from build123d import *

# Parameters (mm, degrees)
F0_R          = 15
F1_DEPTH      = 13
F3_DEPTH      = 25
F3_DEPTH_BACK = 10
F4_R          = 1.5
F5_DEPTH      = 13.001


with BuildPart() as f1:
    # F0 (on Top) → F1 (new body)
    with BuildSketch(Plane.XY):
        Circle(F0_R)
    extrude(amount=F1_DEPTH)

    # F2 (on Right) → F3 (cut, two sides)
    with BuildSketch(Plane.YZ) as f3_sk:
        Polygon((-9, 2), (-9, 0), (9, 0), (9, 2), (10.1, 2), (10.1, 4.1), (-10.1, 4.1), (-10.1, 2), align=None)
    extrude(amount=-F3_DEPTH, mode=Mode.SUBTRACT)
    extrude(f3_sk.sketch, amount=F3_DEPTH_BACK, mode=Mode.SUBTRACT)

    # F4 (on face) → F5 (cut, through all)
    with BuildSketch(Plane.XY.offset(13)):
        Circle(F4_R)
    extrude(amount=-F5_DEPTH, mode=Mode.SUBTRACT)


solid = f1.part
CAD build for the part. Positions are in the model's coordinates, mm. A direction names the side the tool comes from. Round coordinates to 2 decimals unless told otherwise and drop trailing zeros. Order: outer loops, then holes, each group sorted by start corner. A loop starts at its lowest first (then second) coordinate and runs counter-clockwise, first axis right, second up. Notation, with made-up numbers: (-39, 44) - (-30, 44) arc R21 cw to (-30, 69) - close; hole circle Ø6 at (23, -25). An arc over 180 degrees is marked (long way). Return JSON: item names as keys, results as strings.
(1) Cut at C-C (z = 5.25). Give the cut face in (x, y), then the cut area to 3 significant figures.
Answer key:
{"outline": "circle Ø30 at (0, 0); hole circle Ø3 at (0, 0)", "area": "700 mm^2"}
(2) Cut at B-B (x = 0). Give the cut face in (y, z).
Answer key:
{"outline": "(-15, 0) - (-9, 0) - (-9, 2) - (-10.1, 2) - (-10.1, 4.1) - (-1.5, 4.1) - (-1.5, 13) - (-15, 13) - close; (1.5, 4.1) - (10.1, 4.1) - (10.1, 2) - (9, 2) - (9, 0) - (15, 0) - (15, 13) - (1.5, 13) - close"}
(3) Tool access for faces 4 (the face through (-0.8, 9.5, 2)), 5 (the face through (-1, 9, 1)), 6 (the face through (14.307, 4.506, 6.409)): list every direction of +Z, -Z, +X, -X, +Y, -Y with a clear straight run to the whole face (end or side of a thin tool).
Answer key:
{"face 4": "-X", "face 5": "-Z, -X", "face 6": "+Z, -Z"}
(4) Pin check, flat tips, straight feed: pin 1 Ø1.6 at (x, z) = (2, 1) entering from -Y; pin 2 Ø2 at (y, z) = (6.5, 2.5) entering from -X; pin 3 Ø1.5 at (y, z) = (-6, 10.5) entering from -X; pin 4 Ø10 at (x, y) = (3.5, -4.5) entering from -Z. Stop position of each tip, or through.
Answer key:
{"pin 1": "stops at y = -14.95", "pin 2": "stops at x = 10", "pin 3": "stops at x = -14.05", "pin 4": "stops at z = 0"}
(5) Cut at A-A (y = 0). Give the cut face in (x, z), then the cut area to 3 significant figures.
Answer key:
{"outline": "(-15, 4.1) - (-1.5, 4.1) - (-1.5, 13) - (-15, 13) - close; (1.5, 4.1) - (10, 4.1) - (10, 0) - (15, 0) - (15, 13) - (1.5, 13) - close", "area": "261 mm^2"}
(6) Wall check: probe 1 along Y at (x, z) = (0, 6.5); probe 2 along Z at (x, y) = (-11.75, 2.25); probe 3 along Y at (x, z) = (-6, 1.25). Give the ranges that are in metal, low to high. Write a range as from..to.
Answer key:
{"probe 1": "y = -15..-1.5, 1.5..15", "probe 2": "z = 4.1..13", "probe 3": "y = -13.75..-9, 9..13.75"}
(7) Cut at D-D (x = 6.25). Give the cut face in (y, z), then the cut area to 3 significant figures.
Answer key:
{"outline": "(-13.64, 0) - (-9, 0) - (-9, 2) - (-10.1, 2) - (-10.1, 4.1) - (10.1, 4.1) - (10.1, 2) - (9, 2) - (9, 0) - (13.64, 0) - (13.64, 13) - (-13.64, 13) - close", "area": "276 mm^2"}
(8) Pull direction Z, two halves, no side cores. Call faces 1 (the face through (-1.5, 0.07, 8.61)), 2 (the face through (3, 0, 13)), 3 (the face through (0, -10.1, 3)): +Z half, -Z half, draft (parallel to the pull), parting line (faces both ways), or undercut.
Answer key:
{"face 1": "draft", "face 2": "+Z half", "face 3": "undercut"}
